Autodesk Inventor part; units mm, degrees
ref_plane "YZ Plane" through (0, 0, 0) normal (1, 0, 0) x (0, 1, 0)
ref_plane "XZ Plane" through (0, 0, 0) normal (0, 1, 0) x (-1, 0, 0)
ref_plane "XY Plane" through (0, 0, 0) normal (0, 0, 1) x (1, 0, 0)
sketch "スケッチ1" plane through (0, 0, 0) normal (0, 1, 0) x (-1, 0, 0)
  line L0 (25, 25) -> (-25, 25)
  line L1 (-25, 25) -> (-25, -16.9)
  line L2 (-25, -16.9) -> (25, -16.9)
  line L3 (25, -16.9) -> (25, 25)
  circle A0 centre (0, 0) radius 16.5
  point P0 (0, 25)
  dimension "d0" = 50
  dimension "d1" = 16.9
  dimension "d2" = 25
  dimension "d3" = 33
extrude "押し出し1" add sketch "スケッチ1" along normal blind 1.5
sketch "スケッチ2" plane through (0, 1.5, 0) normal (0, 1, 0) x (1, 0, 0)
  line L0 (-11.9569, 9.7901) -> (-18.4521, 13.5401)
  line L1 (-18.4521, 13.5401) -> (-20.9521, 9.2099)
  line L2 (-20.9521, 9.2099) -> (-14.4569, 5.4599)
  line L3 (-14.4569, 5.4599) -> (-11.9569, 9.7901)
  line L4 (-11.9569, 9.7901) -> (-20.9521, 9.2099) construction
  line L5 (-18.4521, 13.5401) -> (-14.4569, 5.4599) construction
  line L6 (20.9521, 9.2099) -> (14.4569, 5.4599)
  line L7 (14.4569, 5.4599) -> (11.9569, 9.7901)
  line L8 (11.9569, 9.7901) -> (18.4521, 13.5401)
  line L9 (18.4521, 13.5401) -> (20.9521, 9.2099)
  line L10 (20.9521, 9.2099) -> (11.9569, 9.7901) construction
  line L11 (14.4569, 5.4599) -> (18.4521, 13.5401) construction
  line L12 (-2.5, -22.75) -> (-2.5, -15.25)
  line L13 (-2.5, -15.25) -> (2.5, -15.25)
  line L14 (2.5, -15.25) -> (2.5, -22.75)
  line L15 (2.5, -22.75) -> (-2.5, -22.75)
  line L16 (-2.5, -22.75) -> (2.5, -15.25) construction
  line L17 (-2.5, -15.25) -> (2.5, -22.75) construction
  line L18 (25, 16.9) -> (-25, 16.9)
  point P0 (0, 0)
  point P1 (0, -19)
  point P2 (-16.4545, 9.5)
  point P3 (16.4545, 9.5)
  dimension "d6" = 120
  dimension "d7" = 120
  dimension "d8" = 19
  dimension "d9" = 19
  dimension "d10" = 19
  dimension "d11" = 30
  dimension "d12" = 30
  dimension "d13" = 5
  dimension "d14" = 7.5
  dimension "d15" = 5
  dimension "d16" = 7.5
  dimension "d17" = 5
  dimension "d18" = 7.5
extrude "押し出し2" cut sketch "スケッチ2" against normal blind 1.5
sketch "スケッチ3" plane through (0, 1.5, 0) normal (0, 1, 0) x (1, 0, 0)
  line L0 (25, -25) -> (25, 16.9)
  line L1 (-25, -25) -> (25, -25)
  line L2 (-25, 16.9) -> (-25, -25)
  line L3 (25, 16.9) -> (-25, 16.9)
  point P0 (0, 0)
  point P1 (-21, -20)
  point P2 (-21, 0)
  point P3 (21, 0)
  point P4 (21, -20)
  dimension "d21" = 4
  dimension "d22" = 5
  dimension "d23" = 4
  dimension "d34" = 20
hole "穴1" at (-21, 1.5, 20) at (-21, 1.5, 0) at (21, 1.5, 0) at (21, 1.5, 20) direction (0, -1, 0) diameter 3 end through all
properties part number "shaft_holder" material "アルミニウム 6061"
Build history of the part. All positions in model axes, mm. A direction names the side the tool comes from. Round coordinates to 2 decimals unless told otherwise and drop trailing zeros. Write each loop counter-clockwise with the first axis right and the second up, starting at its lowest first coordinate (ties: lowest second). Pieces come first, ordered by that corner, then holes.
1) Mould opens along Z. For faces 1 (the flat face through (2.5, 1, 19)), 2 (the flat face through (25, 1, 4)), 3 (the flat face through (0, 1, 25)) say: +Z half, -Z half, draft (parallel to the pull), parting line (faces both ways), or undercut.
2) Drill centre lines: probe 1 along Z at (x, y) = (21, 0.85); probe 2 along X at (y, z) = (0.8, 0); probe 3 along X at (y, z) = (0.55, 20). Where is each one in solid material? Low to high.
3) Band-saw the part on C-C, the plane x = 14.5. List the corners of the cut face in (y, z), and give its area (3 significant figures).
4) Band-saw the part on D-D, the plane z = 7.5. List the corners of the cut face in (x, y), and give its area (3 significant figures).
5) Band-saw the part on A-A, the plane y = 0.3. List the corners of the cut face in (x, z), and give its area (3 significant figures).
6) Band-saw the part on B-B, the plane z = 20. List the corners of the cut face in (x, y), and give its area (3 significant figures).
7) 3-axis set-ups, long thin cutter, end or side, ignore diameter. For faces 4 (the flat face through (6, 0, 18)), 5 (the flat face through (0, 1, 22.75)): which of +Z, -Z, +X, -X, +Y, -Y reach the whole face in a straight line?
Ans:
1. face 1: undercut
1. face 2: draft
1. face 3: +Z half
2. probe 1: z = -16.9 to -1.5, 1.5 to 18.5, 21.5 to 25
2. probe 2: x = -25 to -22.5, -19.5 to -16.5, 16.5 to 19.5, 22.5 to 25
2. probe 3: x = -25 to -22.5, -19.5 to -2.5, 2.5 to 19.5, 22.5 to 25
3. outline: (0, -16.9) - (1.5, -16.9) - (1.5, -11.26) - (0, -11.26) - close; (0, 7.87) - (1.5, 7.87) - (1.5, 25) - (0, 25) - close
3. area: 34.2 mm2
4. outline: (-25, 0) - (-14.7, 0) - (-14.7, 1.5) - (-25, 1.5) - close; (14.7, 0) - (25, 0) - (25, 1.5) - (14.7, 1.5) - close
4. area: 30.9 mm2
5. outline: (-25, -16.9) - (25, -16.9) - (25, 25) - (-25, 25) - close; hole circle Ø3 at (-21, 0); hole circle Ø3 at (-21, 20); hole (-20.95, -9.21) - (-18.45, -13.54) - (-12.87, -10.32) arc R16.5 ccw to (12.87, -10.32) - (18.45, -13.54) - (20.95, -9.21) - (15.37, -5.99) arc R16.5 ccw to (2.5, 16.31) - (2.5, 22.75) - (-2.5, 22.75) - (-2.5, 16.31) arc R16.5 ccw to (-15.37, -5.99) - close; hole circle Ø3 at (21, 0); hole circle Ø3 at (21, 20)
5. area: 1,120 mm2
6. outline: (-25, 0) - (-22.5, 0) - (-22.5, 1.5) - (-25, 1.5) - close; (-19.5, 0) - (-2.5, 0) - (-2.5, 1.5) - (-19.5, 1.5) - close; (2.5, 0) - (19.5, 0) - (19.5, 1.5) - (2.5, 1.5) - close; (22.5, 0) - (25, 0) - (25, 1.5) - (22.5, 1.5) - close
6. area: 58.5 mm2
7. face 4: +Z, -Z, +X, -X, -Y
7. face 5: +Y, -Y
